The figure shows three views and two pictorial views of one solid part (mm, origin at its lowest corner). Answer the questions. Coordinates: 2 decimals unless noted, no trailing zeros. Write each loop counter-clockwise with the first axis right and the second up, starting at its lowest first coordinate (ties: lowest second). Pieces come first, ordered by that corner, then holes. Notation, with made-up numbers: M -34.5,85.25 L 17.5,85.25 A20 ccw 17.5,103.25 Z; hole C 58,-11 d9. An arc over 180 degrees is marked long. Use a Markdown table: item, result. Add a question column.
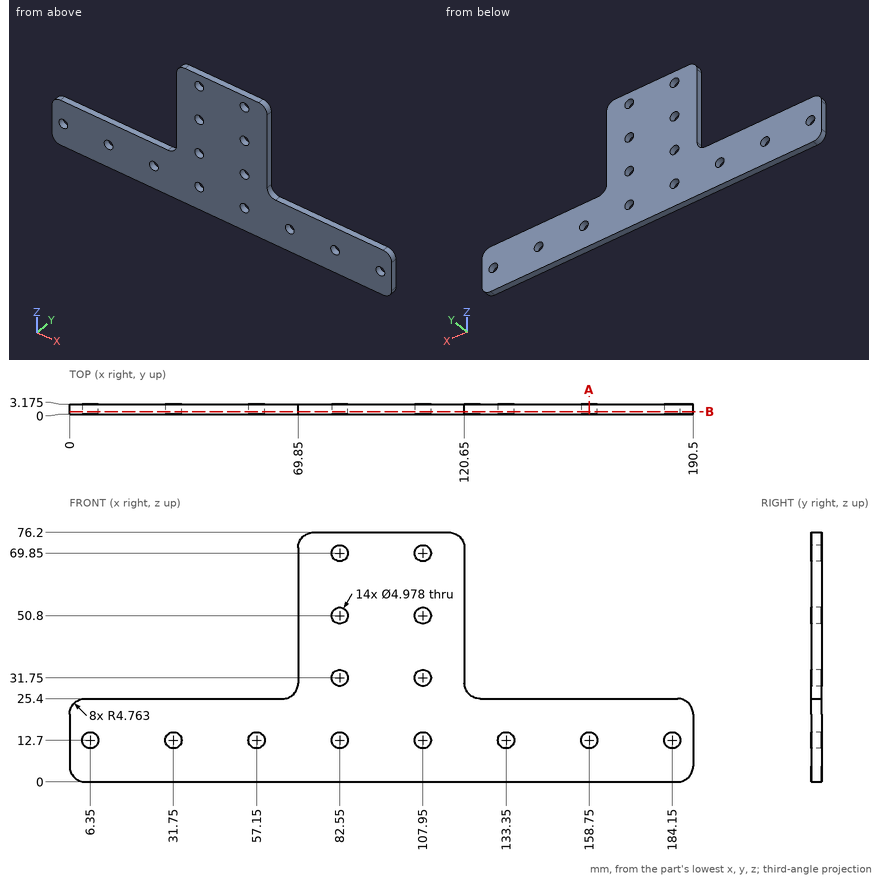
Item 1: Find section B-B on y = 0.85. Count the separate pieces of the cut face and the enclosed holes in it, then the cut area to 3 significant figures.
Item 2: Consider probe 1 along X at (y, z) = (0.85, 31.75); probe 2 along Z at (x, y) = (82.55, 2.35); probe 3 along Z at (x, y) = (6.35, 2.45). Determine where each line is inside the solid, lowest interval first.
Item 3: Each of these flat-tipped pins is pushed along its axis until it touches: pin 1 (6.5 mm diameter, centred on x = 107.95, z = 31.75, fed in from +Y) (1 decimal); pin 2 (1.5 mm diameter, centred on x = 168.5, y = 1.5, fed in from +Z); pin 3 (1 mm diameter, centred on y = 1.5, z = 49.5, fed in from +X). Where does it stop, or does it pass through?
Item 4: Find section A-A on x = 158.75. Give the vertices of the cut face in (y, z) (1 decimal).
Geometry says:
| question | item | result |
|---|---|---|
| 1 | separate pieces | 1 |
| 1 | enclosed holes | 14 |
| 1 | area | 7,130 mm2 |
| 2 | probe 1 | x = 69.85 to 80.06, 85.04 to 105.46, 110.44 to 120.65 |
| 2 | probe 2 | z = 0 to 10.21, 15.19 to 29.26, 34.24 to 48.31, 53.29 to 67.36, 72.34 to 76.2 |
| 2 | probe 3 | z = 0 to 10.21, 15.19 to 25.4 |
| 3 | pin 1 | stops at y = 3.2 |
| 3 | pin 2 | stops at z = 25.4 |
| 3 | pin 3 | stops at x = 120.65 |
| 4 | outline | M 0,0 L 3.2,0 L 3.2,10.2 L 0,10.2 Z; M 0,15.2 L 3.2,15.2 L 3.2,25.4 L 0,25.4 Z |
